Can you work these out from the drawing? Everything is in mm from the part's minimum corner. A direction names the side the tool comes from. Coordinates: 2 decimals unless noted, no trailing zeros. Loops run counter-clockwise (first coordinate to the right, second up) from the corner with the lowest first, then second, coordinate; pieces in that order, holes last.
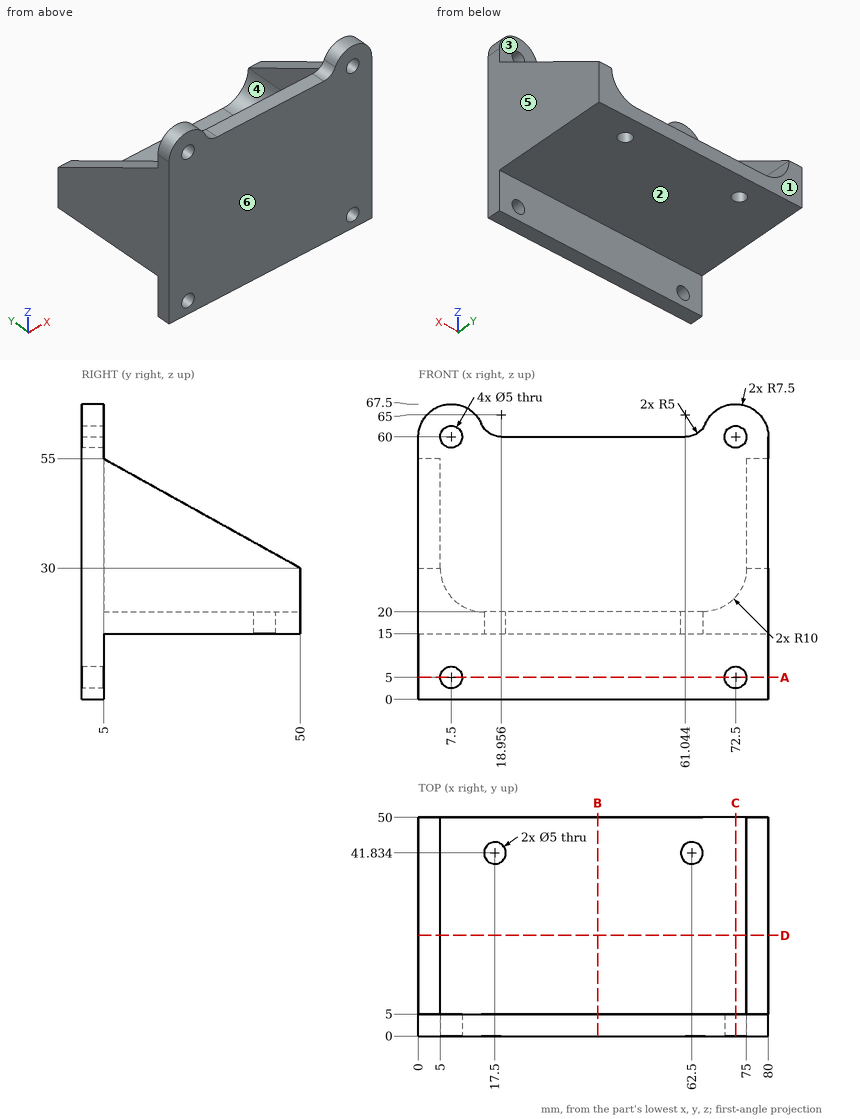
1. On a 3-axis mill with a long thin cutter (end or side, diameter ignored), from which of +Z, -Z, +X, -X, +Y, -Y can I reach the whole of each face in a straight line? I mean the marked faces 1, 2 and 3. Say none if no direction works.
2. I want a section at A-A (z = 5). Please give me the cut outline in (x, y).
3. I need wall thicknesses on line 1 along X through (y, z) = (41, 33); line 2 along X through (y, z) = (3, 5); line 3 along Z through (x, y) = (7, 3). Which ranges of each line are inside material? Lowest first, please.
4. I want a section at D-D (y = 23). Please give me the cut outline in (x, z).
5. I want a section at C-C (x = 72.5). Please give me the cut outline in (y, z) (1 decimal), then the cut area to 3 significant figures.
6. For pin 1 (6 mm diameter, centred on x = 7.5, z = 5, fed in from -Y); pin 2 (22.5 mm diameter, centred on x = 53, y = 36.5, fed in from -Z); pin 3 (2 mm diameter, centred on x = 41.5, z = 26, fed in from +Y); pin 4 (13.5 mm diameter, centred on x = 32, y = 33.5, fed in from +Z), each with a flat end and sliding along its axis, tell me the tip position at first contact or that it passes through.
7. We'd pull the mould along X, two halves only. Please class the marked faces 4, 5 and 6: +X half, -X half, draft (parallel to the pull), parting line (faces both ways), or undercut.
8. I want a section at B-B (x = 41). Please give me the cut outline in (y, z).
Response values:
1. face 1: +Z, -Z, +X, -X, +Y
1. face 2: -Z, +X, -X, +Y
1. face 3: +Z, +Y
2. outline: (0, 0) - (5, 0) - (5, 5) - (0, 5) - close; (10, 0) - (70, 0) - (70, 5) - (10, 5) - close; (75, 0) - (80, 0) - (80, 5) - (75, 5) - close
3. line 1: x = 0 to 5, 75 to 80
3. line 2: x = 0 to 5, 10 to 70, 75 to 80
3. line 3: z = 0 to 2.55, 7.45 to 57.55, 62.45 to 67.48
4. outline: (0, 15) - (80, 15) - (80, 45) - (75, 45) - (75, 30) arc R10 cw to (65, 20) - (15, 20) arc R10 cw to (5, 30) - (5, 45) - (0, 45) - close
5. outline: (0, 0) - (5, 0) - (5, 2.5) - (0, 2.5) - close; (0, 7.5) - (5, 7.5) - (5, 15) - (50, 15) - (50, 23.4) - (5, 23.4) - (5, 57.5) - (0, 57.5) - close; (0, 62.5) - (5, 62.5) - (5, 67.5) - (0, 67.5) - close
5. area: 665 mm2
6. pin 1: stops at y = 0
6. pin 2: stops at z = 15
6. pin 3: stops at y = 5
6. pin 4: stops at z = 20
7. face 4: undercut
7. face 5: +X half
7. face 6: draft
8. outline: (0, 0) - (5, 0) - (5, 15) - (50, 15) - (50, 20) - (5, 20) - (5, 60) - (0, 60) - close
